```python
from build123d import *

# Parameters (mm, degrees)
F2_R           = 1
F3_DEPTH       = 1
F5_D           = 1.6
F5_DEPTH       = 6
F5_CSINK_D     = 3
F5_CSINK_ANGLE = 90
F5_TIP         = 0.4806884952


with BuildPart() as f1:
    # F0 (on Front) → F1 (revolve)
    with BuildSketch(Plane.XZ):
        Polygon((-18, 2.5), (-18, 0), (0, 0), (0, 1.5), align=None)
    revolve(axis=Axis((2.7535289992, 0, 0), (1, 0, 0)))

    # F2 (on Front) → F3 (join, symmetric)
    with BuildSketch(Plane.XZ):
        with BuildLine():
            Line((4.397114317, 2.25), (0, 2.25))
            Line((0, 2.25), (0, -2.25))
            Line((0, -2.25), (4.397114317, -2.25))
            ThreePointArc((4.397114317, -2.25), (5, 0), (4.397114317, 2.25))
        make_face()
        with Locations((2.5, 0)):
            Circle(F2_R, mode=Mode.SUBTRACT)
    extrude(amount=F3_DEPTH, both=True)

    # F5
    with Locations(Plane(origin=(-18, 0, 0), x_dir=(0, -1, 0), z_dir=(-1, 0, 0))):
        with Locations((0, 0)):
            CounterSinkHole(F5_D / 2, F5_CSINK_D / 2, depth=F5_DEPTH, counter_sink_angle=F5_CSINK_ANGLE)
            with Locations((0, 0, -(F5_DEPTH + F5_TIP / 2))):  # 118° drill point
                Cone(0, F5_D / 2, F5_TIP, mode=Mode.SUBTRACT)


solid = f1.part
```
Geometry: final body of the model. Coordinates: model frame, mm. A direction names the side the tool comes from. Coordinates: 2 decimals unless noted, no trailing zeros. Order: outer loops, then holes, each group sorted by start corner. A loop starts at its lowest first (then second) coordinate and runs counter-clockwise, first axis right, second up. Notation, with made-up numbers: (25.5, 25) -> (46.5, 25) arc R17 ccw to (46.5, 46) -> close; hole circle Ø4 at (70.25, 26.25). An arc over 180 degrees is marked (long way). Answer in a Markdown table with one row per item.
Item 1: Draft query along Z for faces 6 (the flat face through (2, 0, 2.25)), 7 (the conical face through (-9, 2, 0)), 8 (the flat face through (0, 0, -2)), 9 (the conical face through (-11.6, 0.11, -0.08)). Return one class per face: released by +Z, released by -Z, zero draft, split by the parting line, or undercut.
Return value:
| item | result |
|---|---|
| face 6 | released by +Z |
| face 7 | split by the parting line |
| face 8 | zero draft |
| face 9 | undercut |
Item 2: Access query for faces 1 (the cylindrical face through (5, 0, 0)), 2 (the cylindrical face through (-14.61, -0.63, -0.49)), 3 (the flat face through (2, 0, -2.25)), 4 (the flat face through (1, -1, 0)), 5 (the flat face through (1, 1, 0)). Directions: +Z, -Z, +X, -X, +Y, -Y. A direction counts if a zero-diameter tool reaches every point of the face in a straight line with its end or side. Return the directions, or none.
Return value:
| item | result |
|---|---|
| face 1 | +X, +Y, -Y |
| face 2 | -X |
| face 3 | -Z, +X, +Y, -Y |
| face 4 | +Z, -Z, +X, -Y |
| face 5 | +Z, -Z, +X, +Y |
Item 3: Section B-B on x = -13. Output: boundary loops of the cut face in (y, z), plus the area to 3 significant figures.
Return value:
| item | result |
|---|---|
| outline | circle Ø4.44 at (0, 0); hole circle Ø1.6 at (0, 0) |
| area | 13.5 mm² |
Item 4: Contact query for flat-ended pins moving along their axis: P1, Ø1.5, axis at x = 0.5, y = -1, coming from the -Z side; P2, Ø2.5, axis at x = 3.5, z = 0.5, coming from the +Y side; P3, Ø1.8, axis at x = 2.5, z = 0, coming from the -Y side; P4, Ø2, axis at x = 3, y = 0, coming from the +Z side. Output: stop coordinate, or through.
Return value:
| item | result |
|---|---|
| P1 | stops at z = -2.25 |
| P2 | stops at y = 1 |
| P3 | passes through |
| P4 | stops at z = 2.25 |
Item 5: Section A-A on x = 2.5. Output: boundary loops of the cut face in (y, z).
Return value:
| item | result |
|---|---|
| outline | (-1, -2.25) -> (1, -2.25) -> (1, -1) -> (-1, -1) -> close; (-1, 1) -> (1, 1) -> (1, 2.25) -> (-1, 2.25) -> close |
Item 6: Ray query, L1, parallel to Z at x = 2.5, y = 0.25; L2, parallel to Z at x = 0.25, y = -0.8; L3, parallel to Y at x = -14.65, z = 0. Return the intervals inside material, ascending.
Return value:
| item | result |
|---|---|
| L1 | z = -2.25 to -1, 1 to 2.25 |
| L2 | z = -2.25 to 2.25 |
| L3 | y = -2.31 to -0.8, 0.8 to 2.31 |
Item 7: Section C-C on x = -5.75. Output: boundary loops of the cut face in (y, z), plus the area to 3 significant figures.
Return value:
| item | result |
|---|---|
| outline | circle Ø3.64 at (0, 0) |
| area | 10.4 mm² |
